Geometry check sheet. Reference: the model listing, model coordinates, mm. A direction names the side the tool comes from. Coordinates: 2 decimals unless noted, no trailing zeros. Write each loop counter-clockwise with the first axis right and the second up, starting at its lowest first coordinate (ties: lowest second). Pieces come first, ordered by that corner, then holes.
from build123d import *

# Parameters (mm, degrees)
SKETCH007_R        = 0.95
PAD003_DEPTH       = 2
PAD004_DEPTH       = 1.2
POLARPATTERN_COUNT = 3
SKETCH013_R        = 2.5
PAD006_DEPTH       = 3.7
SKETCH011_R        = 3.625
SKETCH011_R_2      = 0.5
POCKET003_DEPTH    = 5.701


with BuildPart() as part:
    # Sketch007 (on DatumPlane) → Pad003 (new body)
    with BuildSketch(Plane(origin=(0, 0, -21), x_dir=(1, 0, 0), z_dir=(0, 0, -1))):
        with BuildLine():
            ThreePointArc((22.059707, 1.997961), (11.075, 19.182463), (-9.299569, 20.103247))
            ThreePointArc((-9.299569, 20.103247), (-12.075, 20.914514), (-12.760138, 18.105286))
            ThreePointArc((-12.760138, 18.105286), (-22.15, 0), (-12.760138, -18.105286))
            ThreePointArc((-12.760138, -18.105286), (-12.075, -20.914514), (-9.299569, -20.103247))
            ThreePointArc((-9.299569, -20.103247), (11.075, -19.182463), (22.059707, -1.997961))
            ThreePointArc((22.059707, -1.997961), (24.15, 0), (22.059707, 1.997961))
        make_face()
        with Locations((22.15, 0)):
            Circle(SKETCH007_R, mode=Mode.SUBTRACT)
        with Locations((-11.075, 19.182463)):
            Circle(SKETCH007_R, mode=Mode.SUBTRACT)
        with Locations((-11.075, -19.182463)):
            Circle(SKETCH007_R, mode=Mode.SUBTRACT)
    extrude(amount=PAD003_DEPTH)

    # Sketch008 (on DatumPlane) → Pad004 (join)
    with BuildSketch(Plane.XY.offset(-21)):
        with BuildLine():
            ThreePointArc((20.563616, 3.734664), (10.457001, 18.095887), (-7.03227, 19.681392))
            Line((-7.03227, 19.681392), (-7.008244, 18.41126))
            ThreePointArc((19.172652, 4.527627), (9.229411, 17.404252), (-7.008244, 18.41126))
            ThreePointArc((19.172652, 4.527627), (16.59, 0), (19.172652, -4.527627))
            Line((20.563616, -3.734664), (19.172652, -4.527627))
            ThreePointArc((20.563616, 3.734664), (17.9, 0), (20.563616, -3.734664))
        make_face()
    pad004 = extrude(amount=PAD004_DEPTH)

    # PolarPattern: Pad004 ×3 about axis
    polarpattern_axis = Axis((0, 0, -21), (0, 0, 1))
    for i in range(1, POLARPATTERN_COUNT):
        add(pad004.rotate(polarpattern_axis, i * 360 / POLARPATTERN_COUNT))

    # Sketch013 (on DatumPlane) → Pad006 (join)
    with BuildSketch(Plane.XY.offset(-21)):
        with Locations((-12.02, 8.5)):
            Circle(SKETCH013_R)
        with Locations((-12.02, -8.5)):
            Circle(SKETCH013_R)
    extrude(amount=PAD006_DEPTH)

    # Sketch011 (on DatumPlane) → Pocket003 (cut, through all)
    with BuildSketch(Plane(origin=(0, 0, -23), x_dir=(1, 0, 0), z_dir=(0, 0, -1))):
        with Locations((-12.02, 0)):
            Circle(SKETCH011_R)
        with Locations((-12.02, 8.5)):
            Circle(SKETCH011_R_2)
        with Locations((-12.02, -8.5)):
            Circle(SKETCH011_R_2)
    extrude(amount=-POCKET003_DEPTH, mode=Mode.SUBTRACT)


solid = part.part
1. Sectioned sample at A-A, the plane z = -18.4. Record the boundary of the cut face in (x, y), and give its area (3 significant figures).
Computed values:
outline: circle Ø5 at (-12.02, -8.5); circle Ø5 at (-12.02, 8.5); hole circle Ø1 at (-12.02, -8.5); hole circle Ø1 at (-12.02, 8.5)
area: 37.7 mm2
2. Sectioned sample at B-B, the plane x = -11. Give the number of separate pieces and of enclosed holes in the cut face, and give its area (3 significant figures).
Computed values:
separate pieces: 4
enclosed holes: 0
area: 100 mm2
3. Thickness scan on line 1 along Y through (x, z) = (-12.02, -20.35); line 2 along Y through (x, z) = (-0.5, -20.25); line 3 along Z through (x, y) = (-20, 4.5). Record the ranges inside material, lowest first.
Computed values:
line 1: y = -15.13 to -13.78, -11 to -9, -8 to -6, 6 to 8, 9 to 11, 13.78 to 15.13
line 2: y = -20.89 to -19.69, 19.69 to 20.89
line 3: z = -23 to -19.8
4. Access from +Z, -Z, +X, -X, +Y, -Y to the whole of each face (thin tool, end or side, straight path). Record for faces 1 (the cylindrical face through (10.817, 19.329, -21.986)), 2 (the flat face through (19.968, -3.423, -20.408)), 3 (the cylindrical face through (-8.229, -14.406, -20.408)).
Computed values:
face 1: +Z, -Z, +Y
face 2: +Z, +X
face 3: +Z
5. Draft check along X on faces 4 (the flat face through (-11, -8, -17.3)), 5 (the cylindrical face through (-20.9, 0.26, -20.41)), 6 (the flat face through (-1, 0, -21)). Enter one of: released by +X, released by -X, zero draft, split by the parting line, or undercut.
Computed values:
face 4: zero draft
face 5: released by -X
face 6: undercut
6. Sectioned sample at C-C, the plane y = 17. Record the boundary of the cut face in (x, z), and give its area (3 significant figures).
Computed values:
outline: (-14.2, -23) - (14.2, -23) - (14.2, -21) - (12.16, -21) - (12.16, -19.8) - (9.95, -19.8) - (9.95, -21) - (-6.03, -21) - (-6.03, -19.8) - (-7.47, -19.8) - (-7.47, -21) - (-14.2, -21) - close
area: 61.2 mm2
7. Sectioned sample at D-D, the plane x = -18.5. Record the boundary of the cut face in (y, z), and give its area (3 significant figures).
Computed values:
outline: (-12.18, -23) - (12.18, -23) - (12.18, -21) - (9.72, -21) - (9.72, -19.8) - (6.77, -19.8) - (6.77, -21) - (-6.77, -21) - (-6.77, -19.8) - (-9.72, -19.8) - (-9.72, -21) - (-12.18, -21) - close
area: 55.8 mm2
8. Gauge pin test, flat ends, axial feed: pin 1 Ø3 at (y, z) = (-7, -20.5) entering from -X; pin 2 Ø1.7 at (x, y) = (22.15, 0) entering from +Z; pin 3 Ø4 at (x, y) = (-2.5, -13) entering from +Z; pin 4 Ø3 at (x, z) = (3.5, -20.5) entering from -Y. Record the tip position at first contact, or that the pin passes through.
Computed values:
pin 1: stops at x = -21.43
pin 2: passes through
pin 3: stops at z = -21
pin 4: stops at y = -22.05
